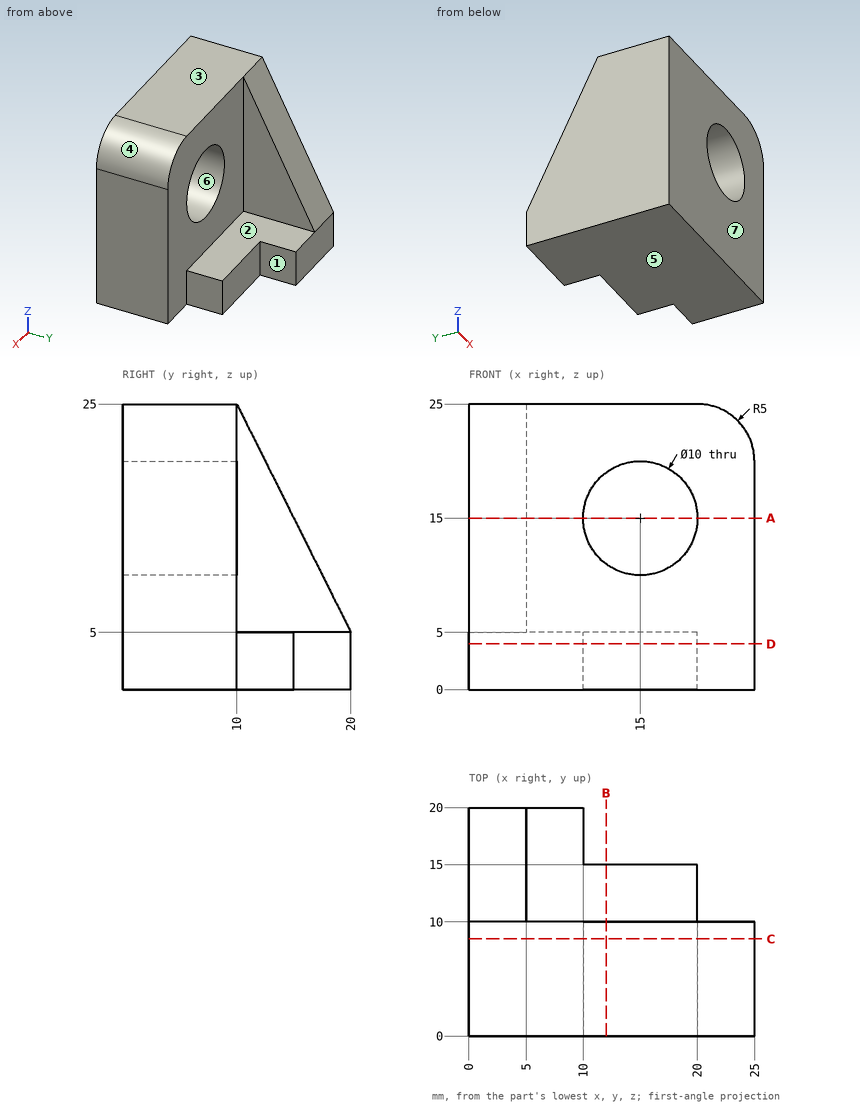
The figure shows three views and two pictorial views of one solid part (mm, origin at its lowest corner). Answer the questions. A direction names the side the tool comes from. Coordinates: 2 decimals unless noted, no trailing zeros. Order: outer loops, then holes, each group sorted by start corner. A loop starts at its lowest first (then second) coordinate and runs counter-clockwise, first axis right, second up.
Q1. Consider line 1 (Z direction, x = 14.75, y = 6); line 2 (X direction, y = 2.5, z = 15); line 3 (Y direction, x = 20.25, z = 13.5). Determine where each line is inside the solid, lowest interval first.
Q2. A cutting plane is placed at B-B, the plane x = 12. Write down the section's boundary in (y, z), and give its area (3 significant figures).
Q3. Given P1, Ø10, axis at y = 16.5, z = 20, coming from the +X side; P2, Ø5, axis at x = 21.5, z = 19.5, coming from the +Y side; P3, Ø8, axis at x = 4.5, y = 15, coming from the +Z side, each flat-ended and moving along its own axis, determine where each tip first touches the part or whether it passes through.
Q4. A cutting plane is placed at A-A, the plane z = 15. Write down the section's boundary in (x, y), and give its area (3 significant figures).
Q5. A cutting plane is placed at C-C, the plane y = 8.5. Write down the section's boundary in (x, z), and give its area (3 significant figures).
Q6. Which of the six approach directions +Z, -Z, +X, -X, +Y, -Y give full straight-line access (tool end or side, diameter ignored) to the marked faces 1, 2 and 3?
Q7. For a pull along Z with two mould halves and no side action, classify the marked faces 4, 5, 6 and 7 as pulls with the +Z half, pulls with the -Z half, needs draft (parallel to the pull), parting line crosses it, or undercut.
Q8. A cutting plane is placed at D-D, the plane z = 4. Write down the section's boundary in (x, y).
Answers follow:
1. line 1: z = 0 to 10.01, 19.99 to 25
1. line 2: x = 0 to 10, 20 to 25
1. line 3: y = 0 to 10
2. outline: (0, 0) - (15, 0) - (15, 5) - (10, 5) - (10, 11) - (0, 11) - close; (0, 19) - (10, 19) - (10, 25) - (0, 25) - close
2. area: 195 mm2
3. P1: stops at x = 5
3. P2: stops at y = 10
3. P3: stops at z = 23
4. outline: (0, 0) - (10, 0) - (10, 10) - (5, 10) - (5, 15) - (0, 15) - close; (20, 0) - (25, 0) - (25, 10) - (20, 10) - close
4. area: 175 mm2
5. outline: (0, 0) - (25, 0) - (25, 20) arc R5 ccw to (20, 25) - (0, 25) - close; hole circle Ø10 at (15, 15)
5. area: 541 mm2
6. face 1: +Z, -Z, +X, +Y
6. face 2: +Z, +X, +Y
6. face 3: +Z, +X, -X, +Y, -Y
7. face 4: pulls with the +Z half
7. face 5: pulls with the -Z half
7. face 6: undercut
7. face 7: needs draft
8. outline: (0, 0) - (25, 0) - (25, 10) - (20, 10) - (20, 15) - (10, 15) - (10, 20) - (0, 20) - close
